Can you work these out from the model? Positions are in its coordinate system, mm. A direction names the side the tool comes from. Give positions to 0.01 mm unless a question says otherwise; leave off trailing zeros. Order: outer loops, then holes, each group sorted by start corner. A loop starts at its lowest first (then second) coordinate and runs counter-clockwise, first axis right, second up. Notation, with made-up numbers: M 17.25,77.5 L 42.25,77.5 A29 ccw 42.25,100.5 Z; hole C 41.25,37.25 d10. An arc over 180 degrees is marked long. One line per question, with ' | ' between items. Start each with the question number.
1) Please list where this line runs through material, in increasing order: line 1 along X through (y, z) = (26.5, 11.5). Write a range as [from, to].
2) If we section it at C-C, the plane x = 46: Please give me the cut outline in (y, z), plus the area to 3 significant figures.
3) If we section it at B-B, the plane y = 5.5: Please give me the cut outline in (x, z), plus the area to 3 significant figures.
4) If we section it at A-A, the plane z = 6.25: Please give me the cut outline in (x, y), plus the area to 3 significant figures.
5) Thinking about a two-plate mould opening in X: for faces 1 (the flat face through (60, 15, 7)), 2 (the flat face through (45, 15, 3)), 3 (the flat face through (23, 30, 7)), which applies, +X half, -X half, draft (parallel to the pull), parting line (faces both ways), or undercut?
6) For faces 4 (the flat face through (40, 15, 8)), 5 (the flat face through (55, 15, 14)), which set-ups out of +Z, -Z, +X, -X, +Y, -Y let a thin tool reach every point of the face, with its end or its side?
```python
from build123d import *

# Parameters (mm, degrees)
BOX001_W     = 40
BOX001_H     = 30
BOX001_DEPTH = 14
BOX002_W     = 10
BOX002_H     = 30
BOX002_DEPTH = 14
BOX_W        = 60
BOX_H        = 30
BOX_DEPTH    = 3


with BuildPart() as cubo001:
    # Box001 → Box001 (new body)
    with BuildSketch(Plane.XY):
        with Locations((20, 15)):
            Rectangle(BOX001_W, BOX001_H)
    extrude(amount=BOX001_DEPTH)


with BuildPart() as cubo002:
    # Box002 → Box002 (new body)
    with BuildSketch(Plane(origin=(50, 0, 0), x_dir=(1, 0, 0), z_dir=(0, 0, 1))):
        with Locations((5, 15)):
            Rectangle(BOX002_W, BOX002_H)
    extrude(amount=BOX002_DEPTH)


with BuildPart() as fusion:
    # Box → Box (new body)
    with BuildSketch(Plane.XY):
        with Locations((30, 15)):
            Rectangle(BOX_W, BOX_H)
    extrude(amount=BOX_DEPTH)

    # Fusion: union Cubo001, Cubo002
    add(cubo001.part)
    add(cubo002.part)


solid = fusion.part
```
Results found:
1) line 1: x = [0, 40], [50, 60]
2) outline: M 0,0 L 30,0 L 30,3 L 0,3 Z | area: 90.0 mm²
3) outline: M 0,0 L 60,0 L 60,14 L 50,14 L 50,3 L 40,3 L 40,14 L 0,14 Z | area: 730 mm²
4) outline: M 0,0 L 40,0 L 40,30 L 0,30 Z; M 50,0 L 60,0 L 60,30 L 50,30 Z | area: 1,500 mm²
5) face 1: +X half | face 2: undercut | face 3: draft
6) face 4: +Z, +Y, -Y | face 5: +Z, +X, -X, +Y, -Y
